Check sheet for the modelled part. Datum: model origin and axes. Units: mm. A direction names the side the tool comes from. Give positions to 0.01 mm unless a question says otherwise; leave off trailing zeros. Order: outer loops, then holes, each group sorted by start corner. A loop starts at its lowest first (then second) coordinate and runs counter-clockwise, first axis right, second up. Notation, with made-up numbers: (-9.75, 74) -> (1.25, 74) arc R17 ccw to (1.25, 94) -> close; hole circle Ø9 at (-39.5, 4). An arc over 180 degrees is marked (long way). Answer in a Markdown table with one row per item. Add a question column.
(1) Cross-section at D-D (y = 300.5). Record the cut outline in (x, z), then the cut area to 3 significant figures.
(2) Set-up check for faces 4 (the face through (13, 103, -3)), 5 (the face through (14.31, 15.23, -1.48)): record each of +Z, -Z, +X, -X, +Y, -Y from which the full face is reachable in a straight line by a thin tool's end or side.
(3) Cross-section at A-A (y = 12.7). Record the cut outline in (x, z).
(4) Release check for a two-part mould opening along X. For faces 1 (the face through (20, 320, -31)), 2 (the face through (-20.27, 193.25, -0.05)), 3 (the face through (12, 103, 0)) record: released by +X, released by -X, zero draft, split by the parting line, or undercut.
(5) Go/stop test with flat-tipped pins: pin 1 (2.5 mm diameter, centred on y = 30.5, z = -1.5, fed in from -X); pin 2 (0.9 mm diameter, centred on x = 21.5, z = -2, fed in from +Y); pin 3 (1 mm diameter, centred on y = 260.5, z = -9.5, fed in from -X). Record where each tip stops, or that it passes through.
(6) Thickness scan on L1, parallel to Z at x = 14, y = 90; L2, parallel to Z at x = 24.5, y = 166.5; L3, parallel to X at y = 148.5, z = 0.5. Record the ranges inside material, lowest first. Write a range as [from, to].
(7) Cross-section at C-C (z = 17). Record the cut outline in (x, y).
(8) Cross-section at B-B (x = 32). Record the cut outline in (y, z), then the cut area to 3 significant figures.
```python
from build123d import *

# Parameters (mm, degrees)
SKETCH1_W           = 3
SKETCH1_H           = 70
BOSS_EXTRUDE1_DEPTH = 25.4
SKETCH2_R           = 3
SKETCH2_R_2         = 1.4
CUT_EXTRUDE1_DEPTH  = 25.4
BOSS_EXTRUDE2_DEPTH = 100
SKETCH4_R           = 33
SKETCH4_R_2         = 30
BOSS_EXTRUDE3_DEPTH = 250


with BuildPart() as part:
    # Sketch1 → Boss-Extrude1 (new body)
    with BuildSketch(Plane(origin=(0, 0, 0), x_dir=(0, 0, -1), z_dir=(1, 0, 0))):
        with Locations((1.5, 35)):
            Rectangle(SKETCH1_W, SKETCH1_H)
    extrude(amount=BOSS_EXTRUDE1_DEPTH)

    # Sketch2 → Cut-Extrude1 (cut)
    with BuildSketch(Plane.XY):
        with Locations((12.7, 12.7)):
            Circle(SKETCH2_R)
        with Locations((12.7, 22.2)):
            Circle(SKETCH2_R_2)
        with Locations((20.927241336, 17.45)):
            Circle(SKETCH2_R_2)
        with Locations((20.927241336, 7.95)):
            Circle(SKETCH2_R_2)
        with Locations((12.7, 3.2)):
            Circle(SKETCH2_R_2)
        with Locations((4.472758664, 7.95)):
            Circle(SKETCH2_R_2)
        with Locations((4.472758664, 17.45)):
            Circle(SKETCH2_R_2)
    extrude(amount=-CUT_EXTRUDE1_DEPTH, mode=Mode.SUBTRACT)

    # Sketch3 → Boss-Extrude2 (add)
    with BuildSketch(Plane(origin=(0, 70, 0), x_dir=(1, 0, 0), z_dir=(0, 1, 0))):
        Polygon((12.7, 0), (42.7, 0), (42.7, 3), (-17.3, 3), (-17.3, 0), align=None)
    extrude(amount=BOSS_EXTRUDE2_DEPTH)

    # Sketch4 → Boss-Extrude3 (add)
    with BuildSketch(Plane.XZ.offset(-70)):
        with Locations((12.7, -1.5)):
            Circle(SKETCH4_R)
        with Locations((12.7, -1.5)):
            Circle(SKETCH4_R_2, mode=Mode.SUBTRACT)
    extrude(amount=-BOSS_EXTRUDE3_DEPTH)


solid = part.part
```
Answer below:
| question | item | result |
|---|---|---|
| 1 | outline | circle Ø66 at (12.7, -1.5); hole circle Ø60 at (12.7, -1.5) |
| 1 | area | 594 mm² |
| 2 | face 4 | +Y, -Y |
| 2 | face 5 | +Z, -Z |
| 3 | outline | (0, -3) -> (9.7, -3) -> (9.7, 0) -> (0, 0) -> close; (15.7, -3) -> (25.4, -3) -> (25.4, 0) -> (15.7, 0) -> close |
| 4 | face 1 | zero draft |
| 4 | face 2 | split by the parting line |
| 4 | face 3 | undercut |
| 5 | pin 1 | stops at x = 0 |
| 5 | pin 2 | stops at y = 170 |
| 5 | pin 3 | stops at x = -19.44 |
| 6 | L1 | z = [-34.47, -31.47], [-3, 0], [28.47, 31.47] |
| 6 | L2 | z = [-32.32, -29.08], [-3, 0], [26.08, 29.32] |
| 6 | L3 | x = [-20.24, -17.23], [42.63, 45.64] |
| 7 | outline | (-14.63, 70) -> (-10.92, 70) -> (-10.92, 320) -> (-14.63, 320) -> close; (36.32, 70) -> (40.03, 70) -> (40.03, 320) -> (36.32, 320) -> close |
| 8 | outline | (70, -28.27) -> (320, -28.27) -> (320, -24.47) -> (70, -24.47) -> close; (70, -3) -> (170, -3) -> (170, 0) -> (70, 0) -> close; (70, 21.47) -> (320, 21.47) -> (320, 25.27) -> (70, 25.27) -> close |
| 8 | area | 2,200 mm² |
